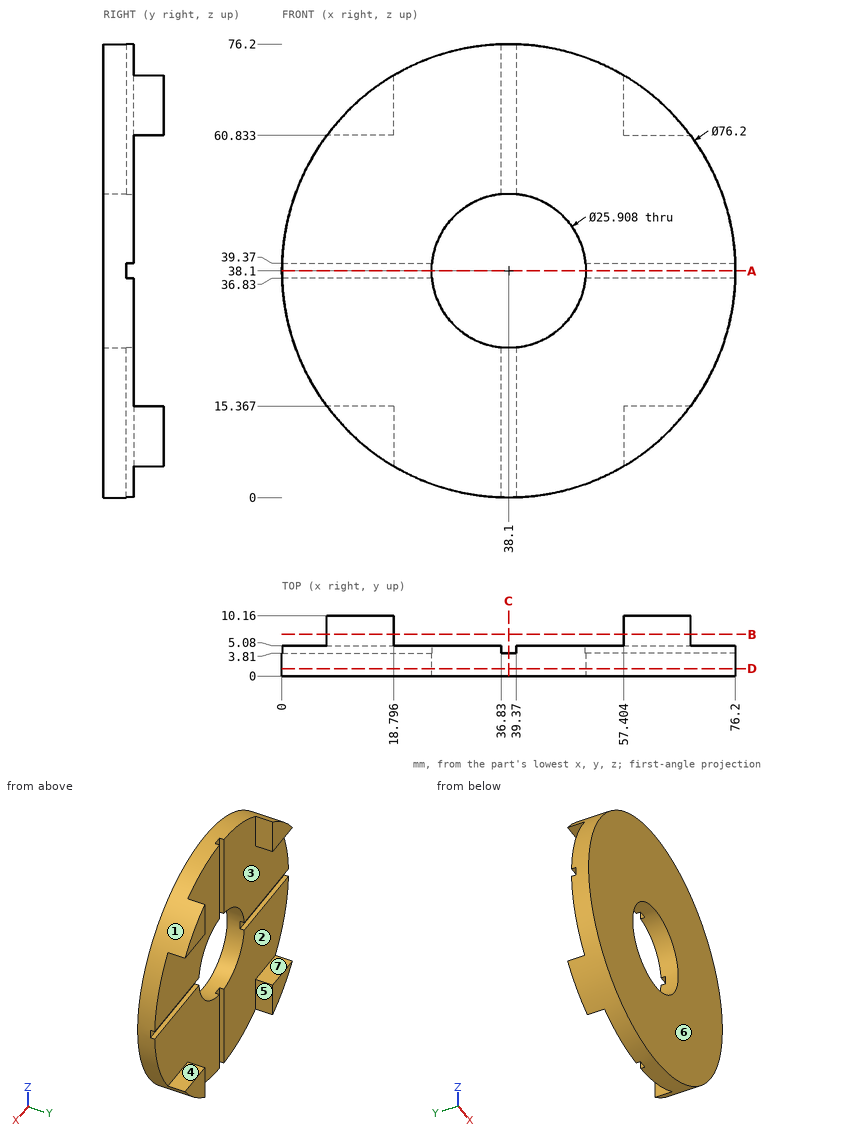
Source: three-view drawing plus pictorial views. Frame: mm from the lowest corner of the part. A direction names the side the tool comes from. Round coordinates to 2 decimals unless told otherwise and drop trailing zeros. Write each loop counter-clockwise with the first axis right and the second up, starting at its lowest first coordinate (ties: lowest second). Pieces come first, ordered by that corner, then holes. Notation, with made-up numbers: M 12,24.5 L 21,24.5 A9 ccw 21,29.5 Z; hole C 86.25,80 d7. An arc over 180 degrees is marked long. Write item = value, one per line.
Item 1: Section query C-C on x = 38.1. Return loops of the section in (y, z).
Findings:
outline = M 0,0 L 3.81,0 L 3.81,25.15 L 0,25.15 Z; M 0,51.05 L 3.81,51.05 L 3.81,76.2 L 0,76.2 Z
Item 2: Section query B-B on y = 7. Return loops of the section in (x, z), then the cut area to 3 significant figures.
Findings:
outline = M 7.53,15.37 A38.1 ccw 18.8,5.25 L 18.8,15.37 Z; M 7.53,60.83 L 18.8,60.83 L 18.8,70.95 A38.1 ccw Z; M 57.4,5.25 A38.1 ccw 68.67,15.37 L 57.4,15.37 Z; M 57.4,60.83 L 68.67,60.83 A38.1 ccw 57.4,70.95 Z
area = 259 mm^2
Item 3: Section query A-A on z = 38.1. Return loops of the section in (x, y), then the cut area to 3 significant figures.
Findings:
outline = M 0,0 L 25.15,0 L 25.15,3.81 L 0,3.81 Z; M 51.05,0 L 76.2,0 L 76.2,3.81 L 51.05,3.81 Z
area = 192 mm^2
Item 4: Pin query (flat end, axial travel): P1, Ø2.5, axis at x = 65.5, y = 9, coming from the +Z side; P2, Ø1, axis at x = 16.5, y = 4.5, coming from the +Z side; P3, Ø5, axis at y = 3, z = 28.5, coming from the +X side; P4, Ø20.5, axis at x = 38.1, z = 38.1, coming from the +Y side. Return the tip coordinate at first contact, or that it passes through.
Findings:
P1 = 65.81
P2 = 69.82
P3 = 75.53
P4 = through
Item 5: Section query D-D on y = 1.25. Return loops of the section in (x, z), then the cut area to 3 significant figures.
Findings:
outline = C 38.1,38.1 d76.2; hole C 38.1,38.1 d25.91
area = 4,030 mm^2
Item 6: Access query for the marked faces 5, 6 and 7. Directions: +Z, -Z, +X, -X, +Y, -Y. A direction counts if a zero-diameter tool reaches every point of the face in a straight line with its end or side. Return the directions, or none.
Findings:
face_5 = +Z, -Z, +Y
face_6 = +Z, -Z, +X, -X, -Y
face_7 = +X, -X, +Y
Item 7: Pull-direction query (X, two-part tool) for the marked faces 1, 2, 3 and 4; classes: pulls with the +X half, pulls with the -X half, needs draft (parallel to the pull), parting line crosses it, or undercut.
Findings:
face_1 = parting line crosses it
face_2 = undercut
face_3 = undercut
face_4 = needs draft
Item 8: Material intervals for line 1 along Z through (x, y) = (38.1, 1.45); line 2 along Y through (x, z) = (62.5, 20), sorted ascending. Write a range as [from, to].
Findings:
line_1 = [0, 25.15], [51.05, 76.2]
line_2 = [0, 5.08]
